from build123d import *

# Parameters (mm, degrees)
SKETCH1_W           = 100
SKETCH1_H           = 63.5
BOSS_EXTRUDE1_DEPTH = 5.08
SKETCH3_W           = 100
SKETCH3_H           = 3.81
BOSS_EXTRUDE2_DEPTH = 19.05
SKETCH8_R           = 4.364936917
CUT_EXTRUDE2_DEPTH  = 84.037054981
SKETCH11_R          = 1.27
CUT_EXTRUDE5_DEPTH  = 64.955604915


with BuildPart() as part:
    # Sketch1 → Boss-Extrude1 (new body)
    with BuildSketch(Plane.XY):
        Rectangle(SKETCH1_W, SKETCH1_H)
    extrude(amount=BOSS_EXTRUDE1_DEPTH)

    # Sketch3 → Boss-Extrude2 (add)
    with BuildSketch(Plane(origin=(0, 0, 0), x_dir=(-1, 0, 0), z_dir=(0, 0, -1))):
        with Locations((0, 29.845)):
            Rectangle(SKETCH3_W, SKETCH3_H)
    extrude(amount=BOSS_EXTRUDE2_DEPTH)

    # Sketch8 → Cut-Extrude2 (cut, through all)
    with BuildSketch(Plane(origin=(0, 31.75, 0), x_dir=(1, 0, 0), z_dir=(0, 1, 0))):
        with Locations(Location((-38.35758865, 8.973092831, 0), (0, 0, 270))):
            Circle(SKETCH8_R)
        with Locations(Location((38.35758865, 8.973092831, 0), (0, 0, 270))):
            Circle(SKETCH8_R)
    extrude(amount=-CUT_EXTRUDE2_DEPTH, mode=Mode.SUBTRACT)

    # Sketch11 → Cut-Extrude5 (cut, through all)
    with BuildSketch(Plane.XY.offset(5.08)):
        with Locations((-43.9547, 15.82674)):
            Circle(SKETCH11_R)
        with Locations((-43.9547, -15.82674)):
            Circle(SKETCH11_R)
        with Locations((43.9547, -15.82674)):
            Circle(SKETCH11_R)
        with Locations((43.9547, 15.82674)):
            Circle(SKETCH11_R)
    extrude(amount=-CUT_EXTRUDE5_DEPTH, mode=Mode.SUBTRACT)


solid = part.part
The listing builds one solid part. Answer for the finished solid, in the listing's coordinates (mm). A direction names the side the tool comes from. Give positions to 0.01 mm unless a question says otherwise; leave off trailing zeros. Loops run counter-clockwise (first coordinate to the right, second up) from the corner with the lowest first, then second, coordinate; pieces in that order, holes last. Notation, with made-up numbers: (7, 23) - (33, 23) arc R23 cw to (33, 33) - close; hole circle Ø3 at (11, 87). An arc over 180 degrees is marked (long way). Answer as a JSON object with one key per item and string values.
1. For a pull along X with two mould halves and no side action, classify faces 3 (the cylindrical face through (43.789, 17.086, 2.576)), 4 (the flat face through (-50, 5, 1)), 5 (the cylindrical face through (-44.12, -14.568, 2.576)), 6 (the flat face through (-1, 0, 5.08)) as pulls with the +X half, pulls with the -X half, needs draft (parallel to the pull), parting line crosses it, or undercut.
Determined:
{"face 3": "undercut", "face 4": "pulls with the -X half", "face 5": "undercut", "face 6": "needs draft"}
2. A cutting plane is placed at B-B (z = -9.5). Write down the section's boundary in (x, y), then the cut area to 3 significant figures.
Determined:
{"outline": "(-50, 27.94) - (-42.69, 27.94) - (-42.69, 31.75) - (-50, 31.75) - close; (-34.02, 27.94) - (34.02, 27.94) - (34.02, 31.75) - (-34.02, 31.75) - close; (42.69, 27.94) - (50, 27.94) - (50, 31.75) - (42.69, 31.75) - close", "area": "315 mm²"}
3. For faces 1 (the cylindrical face through (39.67, 29.87, -4.81)), 2 (the flat face through (-1, -1, 0)), determine the directions among +Z, -Z, +X, -X, +Y, -Y from which every point of the face is accessible in a straight line to the end or side of a thin tool.
Determined:
{"face 1": "+Y, -Y", "face 2": "-Z, +X, -X, -Y"}
4. A cutting plane is placed at D-D (x = -5). Write down the section's boundary in (y, z).
Determined:
{"outline": "(-31.75, 0) - (27.94, 0) - (27.94, -19.05) - (31.75, -19.05) - (31.75, 5.08) - (-31.75, 5.08) - close"}
5. Flat-ended cylindrical pins translate along their axes: pin 1 Ø18 at (x, y) = (-2, -16) entering from -Z; pin 2 Ø1 at (x, z) = (34, -14) entering from -Y; pin 3 Ø12 at (y, z) = (-24.5, -4.5) entering from -X. Find the tip coordinate at first contact, or state that the pin passes through.
Determined:
{"pin 1": "z = 0", "pin 2": "y = 27.94", "pin 3": "x = -50"}
6. A cutting plane is placed at C-C (y = 7.5). Write down the section's boundary in (x, z), then the cut area to 3 significant figures.
Determined:
{"outline": "(-50, 0) - (50, 0) - (50, 5.08) - (-50, 5.08) - close", "area": "508 mm²"}
7. Find the intervals of material crossed by L1, parallel to Z at x = 13.5, y = 26.5; L2, parallel to Y at x = -28.5, z = -3, in increasing order. Write a range as [from, to].
Determined:
{"L1": "[0, 5.08]", "L2": "[27.94, 31.75]"}
8. A cutting plane is placed at A-A (x = 40). Write down the section's boundary in (y, z), then the cut area to 3 significant figures.
Determined:
{"outline": "(-31.75, 0) - (27.94, 0) - (27.94, -4.93) - (31.75, -4.93) - (31.75, 5.08) - (-31.75, 5.08) - close; (27.94, -19.05) - (31.75, -19.05) - (31.75, -13.02) - (27.94, -13.02) - close", "area": "364 mm²"}
